Input: dimensioned drawing with shaded views. Units: mm. Origin: part minimum x, y, z. Round coordinates to 2 decimals unless told otherwise and drop trailing zeros. Order: outer loops, then holes, each group sorted by start corner. A loop starts at its lowest first (then second) coordinate and runs counter-clockwise, first axis right, second up. Notation, with made-up numbers: M 48.25,-24.5 L 77.25,-24.5 A14 cw 77.25,-18.5 Z; hole C 76.5,25 d4. An arc over 180 degrees is marked long. Put each result on its own line as item: value. Start each with the question number.
1) Section C-C, the plane z = 1.1. Return loops of the section in (x, y).
2) Section B-B, the plane x = 144. Return loops of the section in (y, z).
3) Section D-D, the plane y = 93.5. Return loops of the section in (x, z).
4) Section A-A, the plane y = 173. Return loops of the section in (x, z).
5) First-contact query: P1, Ø1.5, axis at x = 140.5, z = 1.5, coming from the -Y side. Flat tip, straight axial feed; report the tip coordinate or a pass-through.
6) Material intervals for probe 1 along X at (y, z) = (92.5, 2.2); probe 2 along Y at (x, z) = (144, 4.2), sorted ascending. Write a range as [from, to].
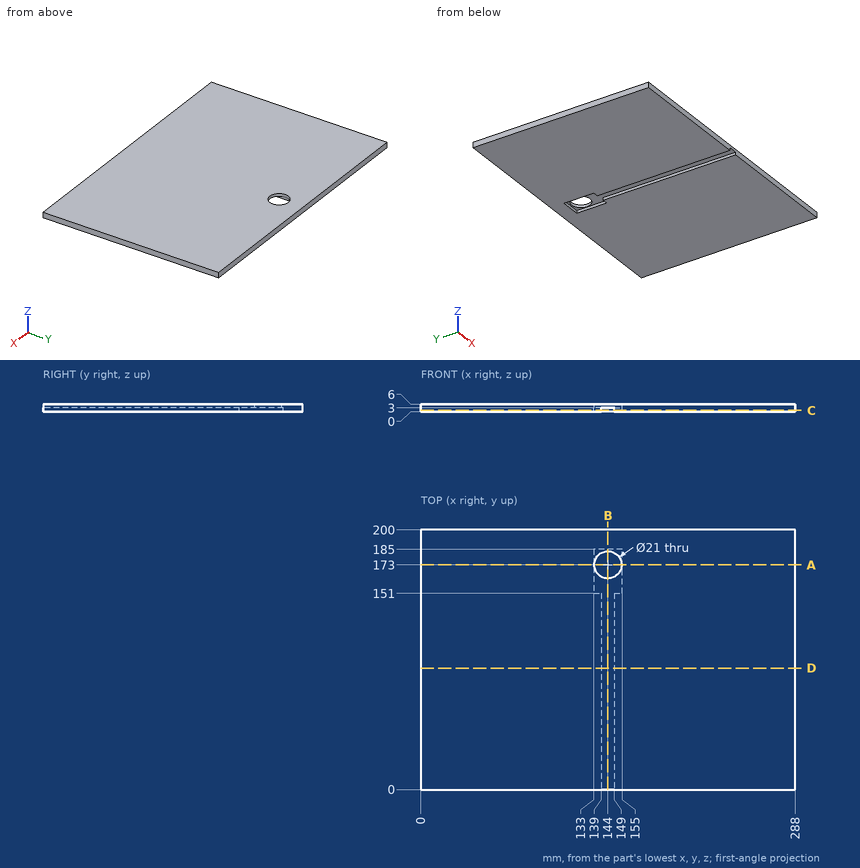
Result sheet:
1. outline: M 0,0 L 139,0 L 139,151 L 133,151 L 133,185 L 155,185 L 155,151 L 149,151 L 149,0 L 288,0 L 288,200 L 0,200 Z
2. outline: M 0,3 L 162.5,3 L 162.5,6 L 0,6 Z; M 183.5,3 L 185,3 L 185,0 L 200,0 L 200,6 L 183.5,6 Z
3. outline: M 0,0 L 139,0 L 139,3 L 149,3 L 149,0 L 288,0 L 288,6 L 0,6 Z
4. outline: M 0,0 L 133,0 L 133,3 L 133.5,3 L 133.5,6 L 0,6 Z; M 154.5,3 L 155,3 L 155,0 L 288,0 L 288,6 L 154.5,6 Z
5. P1: stops at y = 185
6. probe 1: x = [0, 139], [149, 288]
6. probe 2: y = [0, 162.5], [183.5, 200]
